```python
from build123d import *

# Parameters (mm, degrees)
F2_DEPTH = 25.4
F3_DEPTH = 88.646
F4_DEPTH = 310.642
F1_R     = 43.7167010522
F5_DEPTH = 128.016


with BuildPart() as f2:
    # F0 (on Front) → F2 (new body)
    with BuildSketch(Plane.XZ):
        with BuildLine():
            Line((58.3230019719, 0), (0, 0))
            Line((0, 0), (0, -58.3230019719))
            ThreePointArc((0, -58.3230019719), (41.2405901935, -41.2405901935), (58.3230019719, 0))
        make_face()
    extrude(amount=F2_DEPTH)

    # F3 (add): a face of the model
    f3_faces = [f2.faces().sort_by_distance(p)[0] for p in [
        (29.1615009859, -12.7, 0),
    ]]
    extrude(f3_faces, amount=F3_DEPTH)

    # F4 (add): a face of the model
    f4_faces = [f2.faces().sort_by_distance(p)[0] for p in [
        (27.6595840852, -25.4, 20.7894486582),
    ]]
    extrude(f4_faces, amount=F4_DEPTH)

    # F1 (on Front) → F5 (join)
    with BuildSketch(Plane.XZ):
        with Locations((0, -19.1270262003)):
            Circle(F1_R)
    extrude(amount=F5_DEPTH)


solid = f2.part
```
CAD build for the part. Positions are in the model's coordinates, mm. A direction names the side the tool comes from. Coordinates: 2 decimals unless noted, no trailing zeros. Order: outer loops, then holes, each group sorted by start corner. A loop starts at its lowest first (then second) coordinate and runs counter-clockwise, first axis right, second up. Notation, with made-up numbers: (-28.75, 12) -> (19.25, 12) arc R13 ccw to (19.25, 20) -> close; hole circle Ø5 at (-14, -18). An arc over 180 degrees is marked (long way). Use one line per item in the form item = value. Start each with the question number.
1) Tool access for faces 1 (the cylindrical face through (40.785, -165.669, -41.692)), 2 (the flat face through (0, -203, 16)), 3 (the cylindrical face through (-40.454, -63.112, -35.7)): list every direction of +Z, -Z, +X, -X, +Y, -Y with a clear straight run to the whole face (end or side of a thin tool).
2) Drill centre lines: L1, parallel to X at y = -77.5, z = 55.5; L2, parallel to Y at x = -16, z = 10; L3, parallel to Z at x = 1, y = -157. Where is each one in solid material? Low to high. Write a range as [from, to].
3) Band-saw the part on C-C on y = -78. Give the cut face in (x, z).
4) Band-saw the part on B-B on z = 74. Give the cut face in (x, y), then the cut area to 3 significant figures.
5) Band-saw the part on D-D on z = -7.5. Give the cut face in (x, y), then the cut area to 3 significant figures.
6) Band-saw the part on A-A on y = -287. Give the cut face in (x, z), then the cut area to 3 significant figures.
7) Drop flat-ended pins along their axis: pin 1 (12 mm diameter, centred on x = -9, y = -219.5, fed in from +Z); pin 2 (5 mm diameter, centred on y = -127, z = -17, fed in from +X). Give the stop position or say it passes through.
Entries:
q1.face_1 = -Z, +X, -Y
q1.face_2 = +Z, -X, -Y
q1.face_3 = +Y, -Y
q2.L1 = [0, 58.32]
q2.L2 = [-128.02, 0]
q2.L3 = [-58.31, 88.65]
q3.outline = (0, 24.59) arc R43.72 ccw (long way) to (32.36, -48.52) arc R58.32 ccw to (58.32, 0) -> (58.32, 88.65) -> (0, 88.65) -> close
q4.outline = (0, -336.04) -> (58.32, -336.04) -> (58.32, 0) -> (0, 0) -> close
q4.area = 19,600 mm2
q5.outline = (-42.14, -128.02) -> (0, -128.02) -> (0, -336.04) -> (57.84, -336.04) -> (57.84, 0) -> (-42.14, 0) -> close
q5.area = 24,800 mm2
q6.outline = (0, -58.32) arc R58.32 ccw to (58.32, 0) -> (58.32, 88.65) -> (0, 88.65) -> close
q6.area = 7,840 mm2
q7.pin_1 = through
q7.pin_2 = 56.49
